Autodesk Fusion 360 part; units mm, degrees
sketch "Sketch1" plane through (0, 0, 0) normal (0, 0, 1) x (1, 0, 0)
  circle A0 centre (0, 0) radius 2.5
  line L0 (0, 0) -> (5, 8.6603) construction
  line L1 (0, 0) -> (5, -8.6603) construction
  line L2 (0, 0) -> (-5, -8.6603) construction
  line L3 (0, 0) -> (-5, 8.6603) construction
  line L4 (10, 0) -> (-10, 0) construction
  line L5 (2.5981, 4.5) -> (5.1962, 0)
  line L6 (5.1962, 0) -> (2.5981, -4.5)
  line L7 (-2.5981, -4.5) -> (-5.1962, 0)
  line L8 (-5.1962, 0) -> (-2.5981, 4.5)
  line L9 (-2.5981, -4.5) -> (2.5981, -4.5)
  line L10 (-2.5981, 4.5) -> (2.5981, 4.5)
  dimension "d1" = 5
extrude "Extrude1" add sketch "Sketch1" along normal blind 4.5
chamfer "Chamfer1" distance 0.2 angle 45 12 edges at (0, -4.5, 4.5) (-3.8971, -2.25, 4.5) (-3.8971, 2.25, 4.5) (0, 4.5, 4.5) (3.8971, 2.25, 4.5) (3.8971, -2.25, 4.5) (0, -4.5, 0) (-3.8971, -2.25, 0) (-3.8971, 2.25, 0) (0, 4.5, 0) (3.8971, 2.25, 0) (3.8971, -2.25, 0)
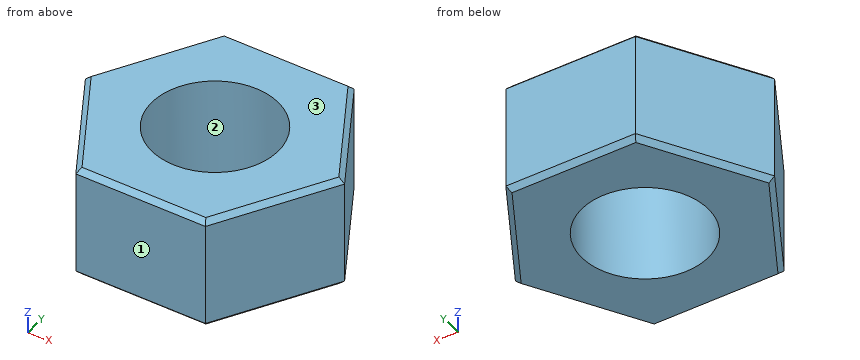
Could you check a few things on this model? Use its own coordinates, in mm. Face numbers are marked on the shaded views. Give positions to 0.01 mm unless a question says otherwise; leave off trailing zeros. Order: outer loops, then holes, each group sorted by start corner. A loop starts at its lowest first (then second) coordinate and runs counter-clockwise, first axis right, second up. Notation, with made-up numbers: (60, -31) - (96, -31) arc R16 cw to (96, -27) - close; hole circle Ø1 at (36.5, 78.5). An arc over 180 degrees is marked (long way). One line per item, written item: value. Start each with the question number.
1. Imagine slicing it at C-C on z = 2.4. List the corners of the cut face in (x, y) for me.
2. Thinking about a two-plate mould opening in Y: for the marked faces 1, 2 and 3, which applies, +Y half, -Y half, draft (parallel to the pull), parting line (faces both ways), or undercut?
3. For P1, Ø1.5, axis at y = -2, z = 1.5, coming from the -X side; P2, Ø4.5, axis at x = 0, y = 0, coming from the -Z side, each with a flat end and sliding along its axis, tell me the tip position at first contact or that it passes through.
4. Imagine slicing it at A-A on x = 0. List the corners of the cut face in (y, z) for me.
5. Imagine slicing it at D-D on y = 3.25. List the corners of the cut face in (x, z) for me, plus the area to 3 significant figures.
6. If I drill on probe 1 along Y at (x, z) = (0, 2.4); probe 2 along X at (y, z) = (-1.75, 2.3); probe 3 along X at (y, z) = (-1, 1.4), over which ranges is the centre line in solid material (lowest first)?
7. Imagine slicing it at B-B on y = -0.25. List the corners of the cut face in (x, z) for me, plus the area to 3 significant figures.
Values:
1. outline: (-5.2, 0) - (-2.6, -4.5) - (2.6, -4.5) - (5.2, 0) - (2.6, 4.5) - (-2.6, 4.5) - close; hole circle Ø5 at (0, 0)
2. face 1: -Y half
2. face 2: undercut
2. face 3: draft
3. P1: x = -4.47
3. P2: through
4. outline: (-4.5, 0.2) - (-4.3, 0) - (-2.5, 0) - (-2.5, 4.5) - (-4.3, 4.5) - (-4.5, 4.3) - close; (2.5, 0) - (4.3, 0) - (4.5, 0.2) - (4.5, 4.3) - (4.3, 4.5) - (2.5, 4.5) - close
5. outline: (-3.32, 0.2) - (-3.09, 0) - (3.09, 0) - (3.32, 0.2) - (3.32, 4.3) - (3.09, 4.5) - (-3.09, 4.5) - (-3.32, 4.3) - close
5. area: 29.8 mm²
6. probe 1: -4.5 to -2.5, 2.5 to 4.5
6. probe 2: -4.19 to -1.79, 1.79 to 4.19
6. probe 3: -4.62 to -2.29, 2.29 to 4.62
7. outline: (-5.05, 0.2) - (-4.82, 0) - (-2.49, 0) - (-2.49, 4.5) - (-4.82, 4.5) - (-5.05, 4.3) - close; (2.49, 0) - (4.82, 0) - (5.05, 0.2) - (5.05, 4.3) - (4.82, 4.5) - (2.49, 4.5) - close
7. area: 23.0 mm²
